For this review, take the finished solid that the model builds, in its own axes (mm). Face numbers are marked on the shaded views. Give positions to 0.01 mm unless a question says otherwise; leave off trailing zeros. Write each loop counter-clockwise with the first axis right and the second up, starting at its lowest first coordinate (ties: lowest second). Pieces come first, ordered by that corner, then holes.
1) We need section B-B on z = 30. Give the boundary of the cut face in (x, y).
2) We need section D-D on x = 31.5. Give the boundary of the cut face in (y, z), and give its area (3 significant figures).
3) For P1, Ø9, axis at x = -95.25, z = -44, coming from the -Y side; P2, Ø6, axis at y = 4, z = -33.5, coming from the +X side; P3, Ø16.5, axis at x = -70.5, y = 24, coming from the +Z side; P4, Ø11.5, axis at x = -102.25, z = 30, coming from the +Y side, all flat-tipped, find the tip position at first contact; note any pin that passes through.
4) Draft analysis for pull direction Z (two halves, no side actions). For the marked faces 1, 2 and 3, state which applies: pulls with the +Z half, pulls with the -Z half, needs draft (parallel to the pull), parting line crosses it, or undercut.
5) We need section C-C on z = -64. Give the boundary of the cut face in (x, y), and give its area (3 significant figures).
6) Wall thickness on line 1 along Z through (x, y) = (106.5, 3.5); line 2 along Z through (x, y) = (55.5, 5.5); line 3 along Y through (x, z) = (21.5, -87): over which ranges is each line inside the solid? List them lowest first.
from build123d import *

# Parameters (mm, degrees)
SKETCH1_W                = 270.5
SKETCH1_H                = 200
MAINBODY_DEPTH           = 9
MAINBODYCURVE_DEPTH      = 100
MAINBODYCURVE_DEPTH_BACK = 100
BOLTHOLE_DEPTH           = 170.097967804
BOLTHOLE_DEPTH_BACK      = 170.097967804
SKETCH5_R                = 5
BOLTHEXHOLE_DEPTH        = 8
SLIDECUT_DEPTH           = 180
SKETCH18_W               = 25
SKETCH18_H               = 5
TABS_DEPTH               = 40
SKETCH19_W               = 15
SKETCH19_H               = 8
TABTRIANGLE1_DEPTH       = 5
TABTRIANGLECUT1_REACH    = 244.128
FILLET1_R                = 10
FILLET2_R                = 5
SKETCH21_W               = 15
SKETCH21_H               = 8
TABTRIANGLE2_DEPTH       = 5
TABTRIANGLECUT2_REACH    = 244.128
FILLET3_R                = 10
FILLET4_R                = 5
CUT_EXTRUDE15_DEPTH      = 173.89465737


with BuildPart() as part:
    # Sketch1 → MainBody (new body)
    with BuildSketch(Plane(origin=(0, 0, 0), x_dir=(1, 0, 0), z_dir=(0, 1, 0))):
        Rectangle(SKETCH1_W, SKETCH1_H)
    extrude(amount=MAINBODY_DEPTH)

    # Sketch12 → MainBodyCurve (add, two sides: drawn at the far end of the back side and taken through both)
    with BuildSketch(Plane.XY.offset(-MAINBODYCURVE_DEPTH_BACK)):
        with BuildLine():
            Line((135.25, 0), (135.25, -7.976686934))
            ThreePointArc((135.25, -7.976686934), (-0.091109356, -7.0779822), (-135.25, 0))
            Line((-135.25, 0), (135.25, 0))
        make_face()
    extrude(amount=MAINBODYCURVE_DEPTH + MAINBODYCURVE_DEPTH_BACK)

    # Sketch5 → BoltHole (cut, two sides: drawn at the far end of the back side and taken through both)
    with BuildSketch(Plane(origin=(0, 9, 0), x_dir=(1, 0, 0), z_dir=(0, 1, 0)).offset(-BOLTHOLE_DEPTH_BACK)):
        with Locations(Location((-102.25, -30, 0), (0, 0, 270))):
            Circle(SKETCH5_R)
        with Locations(Location((-95.25, 44, 0), (0, 0, 270))):
            Circle(SKETCH5_R)
        with Locations(Location((-70.25, 44, 0), (0, 0, 270))):
            Circle(SKETCH5_R)
        with Locations(Location((-62.25, -30, 0), (0, 0, 270))):
            Circle(SKETCH5_R)
    extrude(amount=BOLTHOLE_DEPTH + BOLTHOLE_DEPTH_BACK, mode=Mode.SUBTRACT)

    # Sketch13 → BoltHexHole (cut)
    with BuildSketch(Plane(origin=(0, 9, 0), x_dir=(1, 0, 0), z_dir=(0, 1, 0))):
        Polygon((-87.083976342, 49.445125431), (-95.882605121, 53.794546651), (-104.048628779, 48.34942122), (-103.416023658, 38.554874569), (-94.617394879, 34.205453349), (-86.451371221, 39.65057878), align=None)
        Polygon((-62.430442888, 49.931935595), (-71.477428362, 53.737902903), (-79.296985475, 47.805967308), (-78.069557112, 38.068064405), (-69.022571638, 34.262097097), (-61.203014525, 40.194032692), align=None)
        Polygon((-94.083976342, -24.554874569), (-102.882605121, -20.205453349), (-111.048628779, -25.65057878), (-110.416023658, -35.445125431), (-101.617394879, -39.794546651), (-93.451371221, -34.34942122), align=None)
        Polygon((-54.630390383, -23.813330248), (-63.798008362, -20.307889629), (-71.417617978, -26.494559381), (-69.869609617, -36.186669752), (-60.701991638, -39.692110371), (-53.082382022, -33.505440619), align=None)
    extrude(amount=-BOLTHEXHOLE_DEPTH, mode=Mode.SUBTRACT)

    # Sketch15 → SlideCut (cut)
    with BuildSketch(Plane(origin=(135.25, 0, 0), x_dir=(0, 0, -1), z_dir=(1, 0, 0))):
        Polygon((-85, 14), (85, 14), (85, 4), (95, 4), (95, -1), (-95, -1), (-95, 4), (-85, 4), align=None)
    extrude(amount=-SLIDECUT_DEPTH, mode=Mode.SUBTRACT)

    # Sketch18 → Tabs (add)
    with BuildSketch(Plane(origin=(0, 9, 0), x_dir=(1, 0, 0), z_dir=(0, 1, 0))):
        with Locations((-72.25, -87.5)):
            Rectangle(SKETCH18_W, SKETCH18_H)
        with Locations((-72.25, 87.5)):
            Rectangle(SKETCH18_W, SKETCH18_H)
    extrude(amount=TABS_DEPTH)

    # Sketch19 → TabTriangle1 (add)
    with BuildSketch(Plane(origin=(0, 0, 85), x_dir=(-1, 0, 0), z_dir=(0, 0, -1))):
        with Locations((72.25, 31)):
            Rectangle(SKETCH19_W, SKETCH19_H)
    extrude(amount=TABTRIANGLE1_DEPTH)

    # Sketch20 → TabTriangleCut1 (cut, up to next)
    with BuildSketch(Plane.ZY.offset(79.75), mode=Mode.PRIVATE) as tabtrianglecut1_sk1:
        Polygon((85, 35), (80, 27), (80, 35), align=None)
    tabtrianglecut1_tool1 = extrude(tabtrianglecut1_sk1.sketch, amount=-TABTRIANGLECUT1_REACH, mode=Mode.PRIVATE) & part.part
    add(tabtrianglecut1_tool1.solids().sort_by_distance((-79.75, 32.333333, 81.666667))[0], mode=Mode.SUBTRACT)

    # Fillet1
    fillet1_edges = [part.edges().sort_by_distance(p)[0] for p in [
        (-84.75, 49, 87.5),
        (-59.75, 49, 87.5),
    ]]
    fillet(fillet1_edges, radius=FILLET1_R)

    # Fillet2
    fillet2_edges = [part.edges().sort_by_distance(p)[0] for p in [
        (-84.75, 24, 85),
        (-59.75, 24, 85),
        (-62.678932188, 46.071067812, 85),
        (-72.25, 49, 85),
        (-81.821067812, 46.071067812, 85),
    ]]
    fillet(fillet2_edges, radius=FILLET2_R - 0.0001)  # a hair under: the kernel refuses the full size

    # Sketch21 → TabTriangle2 (add)
    with BuildSketch(Plane.XY.offset(-85)):
        with Locations((-72.25, 31)):
            Rectangle(SKETCH21_W, SKETCH21_H)
    extrude(amount=TABTRIANGLE2_DEPTH)

    # Sketch22 → TabTriangleCut2 (cut, up to next)
    with BuildSketch(Plane.ZY.offset(79.75), mode=Mode.PRIVATE) as tabtrianglecut2_sk1:
        Polygon((-80, 27), (-85, 35), (-80, 35), align=None)
    tabtrianglecut2_tool1 = extrude(tabtrianglecut2_sk1.sketch, amount=-TABTRIANGLECUT2_REACH, mode=Mode.PRIVATE) & part.part
    add(tabtrianglecut2_tool1.solids().sort_by_distance((-79.75, 32.333333, -81.666667))[0], mode=Mode.SUBTRACT)

    # Fillet3
    fillet3_edges = [part.edges().sort_by_distance(p)[0] for p in [
        (-84.75, 49, -87.5),
        (-59.75, 49, -87.5),
    ]]
    fillet(fillet3_edges, radius=FILLET3_R)

    # Fillet4
    fillet4_edges = [part.edges().sort_by_distance(p)[0] for p in [
        (-59.75, 24, -85),
        (-62.678932188, 46.071067812, -85),
        (-72.25, 49, -85),
        (-84.75, 24, -85),
        (-81.821067812, 46.071067812, -85),
    ]]
    fillet(fillet4_edges, radius=FILLET4_R - 0.0001)  # a hair under: the kernel refuses the full size

    # Sketch27 → Cut-Extrude15 (cut, through all)
    with BuildSketch(Plane(origin=(0, 9, 0), x_dir=(1, 0, 0), z_dir=(0, 1, 0))):
        Polygon((-59.75, 100), (-135.25, 70), (-135.25, 100), align=None)
        Polygon((-59.75, -100), (-135.25, -70), (-135.25, -100), align=None)
    extrude(amount=-CUT_EXTRUDE15_DEPTH, mode=Mode.SUBTRACT)


solid = part.part
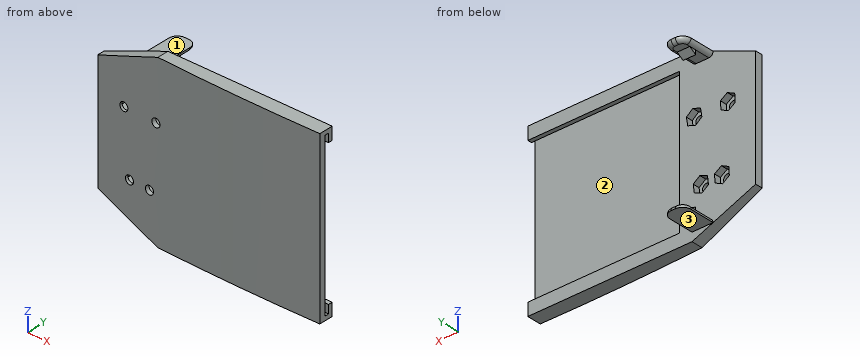
Results list:
1. outline: (-135.25, 0) arc R2963.14 ccw to (-107.25, -1.98) - (-107.25, 1) - (-110.77, 1) - (-110.77, 9) - (-135.25, 9) - close; (-97.25, -2.62) arc R2963.14 ccw to (-67.25, -4.33) - (-67.25, 1) - (-70.86, 1) - (-70.86, 9) - (-93.73, 9) - (-93.73, 1) - (-97.25, 1) - close; (-57.25, -4.84) arc R2963.14 ccw to (135.25, -7.98) - (135.25, -1) - (-44.75, -1) - (-44.75, 9) - (-53.64, 9) - (-53.64, 1) - (-57.25, 1) - close
2. outline: (-7.84, -100) - (9, -100) - (9, -85) - (4, -85) - (4, -95) - (-1, -95) - (-1, 95) - (4, 95) - (4, 85) - (9, 85) - (9, 100) - (-7.84, 100) - close
2. area: 1,570 mm2
3. P1: passes through
3. P2: stops at x = -44.75
3. P3: stops at z = 90
3. P4: stops at y = 1
4. face 1: pulls with the +Z half
4. face 2: undercut
4. face 3: pulls with the -Z half
5. outline: (-135.25, 0) arc R2963.14 ccw to (135.25, -7.98) - (135.25, -1) - (-44.75, -1) - (-44.75, 9) - (-135.25, 9) - close
5. area: 2,270 mm2
6. line 1: z = -100 to -95, 95 to 100
6. line 2: z = -100 to -85, 85 to 100
6. line 3: y = -7.64 to -1, 4 to 9
